from build123d import *

# Parameters (mm, degrees)
SCHIZZO1_R                   = 25
ESTRUSIONE_ESTRUSIONE1_DEPTH = 5
SCHIZZO2_R                   = 20
ESTRUSIONE_ESTRUSIONE2_DEPTH = 5
SCHIZZO3_R                   = 15
ESTRUSIONE_ESTRUSIONE3_DEPTH = 5
SCHIZZO4_R                   = 10
ESTRUSIONE_ESTRUSIONE4_DEPTH = 5
SCHIZZO6_R                   = 30
ESTRUSIONE_ESTRUSIONE6_DEPTH = 5


with BuildPart() as part:
    # Schizzo1 → Estrusione-Estrusione1 (new body)
    with BuildSketch(Plane(origin=(0, 0, 0), x_dir=(1, 0, 0), z_dir=(0, 1, 0))):
        with Locations(Location((0, 0, 0), (0, 0, 270))):
            Circle(SCHIZZO1_R)
    extrude(amount=ESTRUSIONE_ESTRUSIONE1_DEPTH)

    # Schizzo2 → Estrusione-Estrusione2 (add)
    with BuildSketch(Plane(origin=(0, 5, 0), x_dir=(1, 0, 0), z_dir=(0, 1, 0))):
        with Locations(Location((0, 0, 0), (0, 0, 270))):
            Circle(SCHIZZO2_R)
    extrude(amount=ESTRUSIONE_ESTRUSIONE2_DEPTH)

    # Schizzo3 → Estrusione-Estrusione3 (add)
    with BuildSketch(Plane(origin=(0, 10, 0), x_dir=(1, 0, 0), z_dir=(0, 1, 0))):
        with Locations(Location((0, 0, 0), (0, 0, 270))):
            Circle(SCHIZZO3_R)
    extrude(amount=ESTRUSIONE_ESTRUSIONE3_DEPTH)

    # Schizzo4 → Estrusione-Estrusione4 (add)
    with BuildSketch(Plane(origin=(0, 15, 0), x_dir=(1, 0, 0), z_dir=(0, 1, 0))):
        with Locations(Location((0, 0, 0), (0, 0, 270))):
            Circle(SCHIZZO4_R)
    extrude(amount=ESTRUSIONE_ESTRUSIONE4_DEPTH)

    # Schizzo6 → Estrusione-Estrusione6 (add)
    with BuildSketch(Plane.XZ):
        with Locations(Location((0, 0, 0), (0, 0, 270))):
            Circle(SCHIZZO6_R)
    extrude(amount=ESTRUSIONE_ESTRUSIONE6_DEPTH)


solid = part.part
Source: CAD feature listing. Evaluate the final solid. Frame: model axes, mm. A direction names the side the tool comes from. Round coordinates to 2 decimals unless told otherwise and drop trailing zeros. Order: outer loops, then holes, each group sorted by start corner. A loop starts at its lowest first (then second) coordinate and runs counter-clockwise, first axis right, second up. Notation, with made-up numbers: (32, -37) - (55, -37) arc R16 cw to (55, -27) - close; hole circle Ø1 at (-34, -34). An arc over 180 degrees is marked (long way). Use a Markdown table: item, result. Add a question column.
1. Set-up query: faces 1 (the flat face through (0, -5, 0)), 2 (the flat face through (15, 10, 3)). Return all of +Z, -Z, +X, -X, +Y, -Y with unobstructed straight access to the full face (end or side cutting, diameter ignored); none if empty.
2. Section query D-D (x = 0). Return the cut outline in (y, z).
3. Line query: probe 1 along Y at (x, z) = (15, -9.5); probe 2 along Y at (x, z) = (-21, -9); probe 3 along Z at (x, y) = (-26.5, -1.25). Output: solid intervals per line, ascending.
4. Section query A-A (z = 0). Return the cut outline in (x, y).
5. Section query B-B (x = 24). Return the cut outline in (y, z).
6. Section query C-C (y = 6.25). Return the cut outline in (x, z), then the cut area to 3 significant figures.
7. First-contact query: pin 1 (5 mm diameter, centred on y = 11, z = -11.5, fed in from -X); pin 2 (8 mm diameter, centred on y = 3, z = 15.5, fed in from -X); pin 3 (12 mm diameter, centred on y = 12.5, z = -9, fed in from +X); pin 4 (6 mm diameter, centred on x = 7.5, z = 7.5, fed in from +Y). Flat tips, straight axial feed; report the tip coordinate or a pass-through.
Derived:
| question | item | result |
|---|---|---|
| 1 | face 1 | +Z, -Z, +X, -X, -Y |
| 1 | face 2 | +Y |
| 2 | outline | (-5, -30) - (0, -30) - (0, -25) - (5, -25) - (5, -20) - (10, -20) - (10, -15) - (15, -15) - (15, -10) - (20, -10) - (20, 10) - (15, 10) - (15, 15) - (10, 15) - (10, 20) - (5, 20) - (5, 25) - (0, 25) - (0, 30) - (-5, 30) - close |
| 3 | probe 1 | -5 to 10 |
| 3 | probe 2 | -5 to 5 |
| 3 | probe 3 | -14.06 to 14.06 |
| 4 | outline | (-30, -5) - (30, -5) - (30, 0) - (25, 0) - (25, 5) - (20, 5) - (20, 10) - (15, 10) - (15, 15) - (10, 15) - (10, 20) - (-10, 20) - (-10, 15) - (-15, 15) - (-15, 10) - (-20, 10) - (-20, 5) - (-25, 5) - (-25, 0) - (-30, 0) - close |
| 5 | outline | (-5, -18) - (0, -18) - (0, -7) - (5, -7) - (5, 7) - (0, 7) - (0, 18) - (-5, 18) - close |
| 6 | outline | circle Ø40 at (0, 0) |
| 6 | area | 1,260 mm2 |
| 7 | pin 1 | x = -17.75 |
| 7 | pin 2 | x = -27.11 |
| 7 | pin 3 | x = 19.68 |
| 7 | pin 4 | y = 20 |
